from build123d import *

# Parameters (mm, degrees)
SKETCH_W        = 50
SKETCH_H        = 30
PAD_DEPTH       = 15
SKETCH002_W     = 44
SKETCH002_H     = 24
POCKET_DEPTH    = 12
SKETCH003_W     = 52.437362
SKETCH003_H     = 33.156771
SKETCH003_W_2   = 46.5
SKETCH003_H_2   = 26.5
POCKET001_DEPTH = 7


with BuildPart() as part:
    # Sketch → Pad (new body)
    with BuildSketch(Plane.XY):
        Rectangle(SKETCH_W, SKETCH_H)
    extrude(amount=PAD_DEPTH)

    # Sketch002 (on Face6 of Pad) → Pocket (cut)
    with BuildSketch(Plane.XY.offset(15)):
        Rectangle(SKETCH002_W, SKETCH002_H)
    extrude(amount=-POCKET_DEPTH, mode=Mode.SUBTRACT)

    # Sketch003 (on Face5 of Pocket) → Pocket001 (cut)
    with BuildSketch(Plane.XY.offset(15)):
        with Locations((-0.04809, 0.412657)):
            Rectangle(SKETCH003_W, SKETCH003_H)
        with Locations((0.272907, 0)):
            Rectangle(SKETCH003_W_2, SKETCH003_H_2, mode=Mode.SUBTRACT)
    extrude(amount=-POCKET001_DEPTH, mode=Mode.SUBTRACT)


solid = part.part
Can you work these out from the model? Positions are in its coordinate system, mm. A direction names the side the tool comes from. Coordinates: 2 decimals unless noted, no trailing zeros. Write each loop counter-clockwise with the first axis right and the second up, starting at its lowest first coordinate (ties: lowest second). Pieces come first, ordered by that corner, then holes. Notation, with made-up numbers: (75, 44.5) -> (133, 44.5) arc R11 ccw to (133, 58.5) -> close; hole circle Ø11 at (-33, 79.25). An arc over 180 degrees is marked (long way). Answer as CSV lines item,"result".
1) If we section it at B-B on y = 6.25: Please give me the cut outline in (x, z), then the cut area to 4 significant figures.
Check result:
outline,"(-25, 0) -> (25, 0) -> (25, 8) -> (23.52, 8) -> (23.52, 15) -> (22, 15) -> (22, 3) -> (-22, 3) -> (-22, 15) -> (-22.98, 15) -> (-22.98, 8) -> (-25, 8) -> close"
area,"197.5 mm²"
2) If I drill on line 1 (Y direction, x = -20, z = 14.25); line 2 (Y direction, x = -14, z = 4.25); line 3 (X direction, y = 4, z = 3.25), over which ranges is the centre line in solid material (lowest first)? Write a range as from..to.
Check result:
line 1,"-13.25..-12, 12..13.25"
line 2,"-15..-12, 12..15"
line 3,"-25..-22, 22..25"
3) If we section it at D-D on z = 7.5: Please give me the cut outline in (x, y), then the cut area to 3 significant figures.
Check result:
outline,"(-25, -15) -> (25, -15) -> (25, 15) -> (-25, 15) -> close; hole (-22, -12) -> (22, -12) -> (22, 12) -> (-22, 12) -> close"
area,"444 mm²"
4) If we section it at A-A on z = 13.25: Please give me the cut outline in (x, y).
Check result:
outline,"(-22.98, -13.25) -> (23.52, -13.25) -> (23.52, 13.25) -> (-22.98, 13.25) -> close; hole (-22, -12) -> (22, -12) -> (22, 12) -> (-22, 12) -> close"
5) If we mould it in two halves opening along X, with no side actions, what happens to faces 4 (the flat face through (23.523, 0, 12)), 5 (the flat face through (-25, 0, 4)), 6 (the flat face through (0, -14, 8)), 7 (the flat face through (0, 12, 9))? For each: +X half, -X half, draft (parallel to the pull), parting line (faces both ways), or undercut.
Check result:
face 4,"+X half"
face 5,"-X half"
face 6,"draft"
face 7,"undercut"
6) Will these pins go through, and if not, where does the flat tip stop? P1, Ø3.5, axis at y = -4.5, z = 13, coming from the -X side; P2, Ø7.5, axis at x = -8, z = 12.5, coming from the +Y side; P3, Ø5.5, axis at y = 0.5, z = 12.5, coming from the +X side.
Check result:
P1,"x = -22.98"
P2,"y = 13.25"
P3,"x = 23.52"
7) If we section it at C-C on x = -16: Please give me the cut outline in (y, z), then the cut area to 4 significant figures.
Check result:
outline,"(-15, 0) -> (15, 0) -> (15, 8) -> (13.25, 8) -> (13.25, 15) -> (12, 15) -> (12, 3) -> (-12, 3) -> (-12, 15) -> (-13.25, 15) -> (-13.25, 8) -> (-15, 8) -> close"
area,"137.5 mm²"
8) On a 3-axis mill with a long thin cutter (end or side, diameter ignored), from which of +Z, -Z, +X, -X, +Y, -Y can I reach the whole of each face in a straight line? I mean faces 1 (the flat face through (22, 0, 9)), 2 (the flat face through (-22.977, 0, 12)), 3 (the flat face through (0, -13.25, 12)). Say none if no direction works.
Check result:
face 1,"+Z"
face 2,"+Z, -X, +Y, -Y"
face 3,"+Z, +X, -X, -Y"
